```python
from build123d import *

# Parameters (mm, degrees)
SKETCH2_W           = 50
SKETCH2_H           = 50
SKETCH2_R           = 22.5
SKETCH2_R_2         = 14.5
SKETCH2_R_3         = 2.75
BOSS_EXTRUDE1_DEPTH = 10
SKETCH2_3_R         = 22.5
SKETCH2_3_R_2       = 14.5
SKETCH2_3_R_3       = 2.75
BOSS_EXTRUDE2_DEPTH = 40
SKETCH2_4_R         = 14.5
SKETCH2_4_R_2       = 2.75
BOSS_EXTRUDE3_DEPTH = 41
SKETCH2_5_R         = 2.75
BOSS_EXTRUDE4_DEPTH = 55
SKETCH4_R           = 1.6
CUT_EXTRUDE1_DEPTH  = 66.383484153


with BuildPart() as part:
    # Sketch2 → Boss-Extrude1 (new body)
    # profile 1 of 4: a face of its own
    with BuildSketch(Plane.XY):
        Rectangle(SKETCH2_W, SKETCH2_H)
        Circle(SKETCH2_R, mode=Mode.SUBTRACT)
    # profile 2 of 4: a face of its own
    with BuildSketch(Plane.XY):
        Circle(SKETCH2_R)
        Circle(SKETCH2_R_2, mode=Mode.SUBTRACT)
    # profile 3 of 4: a face of its own
    with BuildSketch(Plane.XY):
        Circle(SKETCH2_R_2)
        Circle(SKETCH2_R_3, mode=Mode.SUBTRACT)
    # profile 4 of 4: a face of its own
    with BuildSketch(Plane.XY):
        Circle(SKETCH2_R_3)
    extrude(amount=BOSS_EXTRUDE1_DEPTH)

    # Sketch2_3 → Boss-Extrude2 (add)
    # profile 1 of 3: a face of its own
    with BuildSketch(Plane.XY):
        Circle(SKETCH2_3_R)
        Circle(SKETCH2_3_R_2, mode=Mode.SUBTRACT)
    # profile 2 of 3: a face of its own
    with BuildSketch(Plane.XY):
        Circle(SKETCH2_3_R_2)
        Circle(SKETCH2_3_R_3, mode=Mode.SUBTRACT)
    # profile 3 of 3: a face of its own
    with BuildSketch(Plane.XY):
        Circle(SKETCH2_3_R_3)
    extrude(amount=BOSS_EXTRUDE2_DEPTH)

    # Sketch2_4 → Boss-Extrude3 (add)
    with BuildSketch(Plane.XY):
        Circle(SKETCH2_4_R)
        Circle(SKETCH2_4_R_2, mode=Mode.SUBTRACT)
    extrude(amount=BOSS_EXTRUDE3_DEPTH)

    # Sketch2_5 → Boss-Extrude4 (add)
    with BuildSketch(Plane.XY):
        Circle(SKETCH2_5_R)
    extrude(amount=BOSS_EXTRUDE4_DEPTH)

    # Sketch4 → Cut-Extrude1 (cut, through all)
    with BuildSketch(Plane(origin=(0, 0, 0), x_dir=(-1, 0, 0), z_dir=(0, 0, -1))):
        with Locations((-21.5, 21.5)):
            Circle(SKETCH4_R)
        with Locations(Location((-21.5, -21.5, 0), (0, 0, 180))):
            Circle(SKETCH4_R)
        with Locations((21.5, -21.5)):
            Circle(SKETCH4_R)
        with Locations(Location((21.5, 21.5, 0), (0, 0, 180))):
            Circle(SKETCH4_R)
    extrude(amount=-CUT_EXTRUDE1_DEPTH, mode=Mode.SUBTRACT)


solid = part.part
```
Check sheet for the modelled part. Datum: model origin and axes. Units: mm. A direction names the side the tool comes from. Give positions to 0.01 mm unless a question says otherwise; leave off trailing zeros. Order: outer loops, then holes, each group sorted by start corner. A loop starts at its lowest first (then second) coordinate and runs counter-clockwise, first axis right, second up. Notation, with made-up numbers: M -20.75,3 L 11.25,3 A26 ccw 11.25,28 Z; hole C 15,-15 d3. An arc over 180 degrees is marked long. Answer in a Markdown table with one row per item.
1) Access from +Z, -Z, +X, -X, +Y, -Y to the whole of each face (thin tool, end or side, straight path). Record for faces 4 (the cylindrical face through (-21.292, -19.914, 4.93)), 5 (the flat face through (0, -15, 40)).
Filled sheet:
| item | result |
|---|---|
| face 4 | +Z, -Z |
| face 5 | +Z |
2) Cross-section at B-B, the plane x = 0. Enter the section's corners in (y, z), plus the area to 3 significant figures.
Filled sheet:
| item | result |
|---|---|
| outline | M -25,0 L 25,0 L 25,10 L 22.5,10 L 22.5,40 L 14.5,40 L 14.5,41 L 2.75,41 L 2.75,55 L -2.75,55 L -2.75,41 L -14.5,41 L -14.5,40 L -22.5,40 L -22.5,10 L -25,10 Z |
| area | 1,960 mm2 |
3) Gauge pin test, flat ends, axial feed: P1, Ø3, axis at x = 12.5, y = -11.5, coming from the -Z side; P2, Ø4, axis at y = 12, z = 24, coming from the +X side; P3, Ø1.5, axis at y = 6.5, z = 33, coming from the -X side; P4, Ø8, axis at x = 12, z = 21.5, coming from the -Y side. Record the tip position at first contact, or that the pin passes through.
Filled sheet:
| item | result |
|---|---|
| P1 | stops at z = 0 |
| P2 | stops at x = 20.16 |
| P3 | stops at x = -21.75 |
| P4 | stops at y = -21.03 |
4) Release check for a two-part mould opening along Y. For faces 1 (the flat face through (0, 0, 0)), 2 (the cylindrical face through (-21.708, 19.914, 4.93)), 3 (the flat face through (0, 25, 5)) record: +Y half, -Y half, draft (parallel to the pull), parting line (faces both ways), or undercut.
Filled sheet:
| item | result |
|---|---|
| face 1 | draft |
| face 2 | undercut |
| face 3 | +Y half |
5) Cross-section at A-A, the plane y = 21.5. Enter the section's corners in (x, z).
Filled sheet:
| item | result |
|---|---|
| outline | M -25,0 L -23.1,0 L -23.1,10 L -25,10 Z; M -19.9,0 L 19.9,0 L 19.9,10 L 6.63,10 L 6.63,40 L -6.63,40 L -6.63,10 L -19.9,10 Z; M 23.1,0 L 25,0 L 25,10 L 23.1,10 Z |
6) Thickness scan on L1, parallel to Y at x = -21.5, z = 4; L2, parallel to X at y = -21, z = 5; L3, parallel to Z at x = -8.5, y = 3. Record the ranges inside material, lowest first. Write a range as [from, to].
Filled sheet:
| item | result |
|---|---|
| L1 | y = [-25, -23.1], [-19.9, 19.9], [23.1, 25] |
| L2 | x = [-25, -23.02], [-19.98, 19.98], [23.02, 25] |
| L3 | z = [0, 41] |
